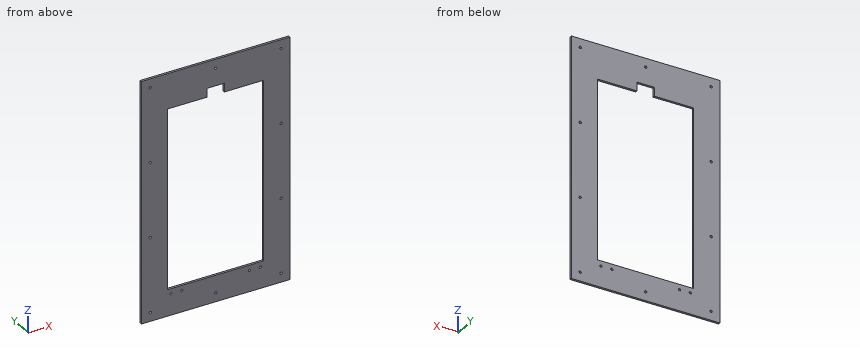
Autodesk Inventor part; units mm, degrees
ref_plane "YZ Plane" through (0, 0, 0) normal (1, 0, 0) x (0, 1, 0)
ref_plane "XZ Plane" through (0, 0, 0) normal (0, 1, 0) x (-1, 0, 0)
ref_plane "XY Plane" through (0, 0, 0) normal (0, 0, 1) x (1, 0, 0)
sketch "Sketch1" plane through (0, 0, 0) normal (0, 1, 0) x (-1, 0, 0)
  line L0 (107.95, -174.625) -> (-107.95, -174.625)
  line L1 (-107.95, -174.625) -> (-107.95, 174.625)
  line L2 (-107.95, 174.625) -> (107.95, 174.625)
  line L3 (107.95, 174.625) -> (107.95, -174.625)
  line L4 (107.95, -174.625) -> (-107.95, 174.625) construction
  line L5 (-107.95, -174.625) -> (107.95, 174.625) construction
  point P0 (0, 0)
  dimension "d0" = 215.9
  dimension "d1" = 349.25
extrude "Thickness" add sketch "Sketch1" along normal blind 3.175
sketch "Cutout Sketch" plane through (0, 3.175, 0) normal (0, 1, 0) x (1, 0, 0)
  line L0 (107.95, -174.625) -> (107.95, 174.625)
  line L1 (107.95, 174.625) -> (-107.95, 174.625)
  line L2 (-107.95, 174.625) -> (-107.95, -174.625)
  line L3 (-107.95, -174.625) -> (107.95, -174.625)
  line L4 (-69.85, 136.525) -> (69.85, 136.525)
  line L5 (69.85, 136.525) -> (69.85, -123.825)
  line L6 (69.85, -123.825) -> (-69.85, -123.825)
  line L7 (-69.85, -123.825) -> (-69.85, 136.525)
  point P0 (0, 0)
  dimension "d4" = 38.1
  dimension "d8" = 38.1
  dimension "d9" = 50.8
  dimension "d10" = 38.1
extrude "Cutout" cut sketch "Cutout Sketch" against normal blind 25.4 contours L4 L5 L6 L7
sketch "Sketch3" plane through (0, 3.175, 0) normal (0, 1, 0) x (1, 0, 0)
  line L0 (69.85, 136.525) -> (69.85, -123.825)
  line L1 (69.85, -123.825) -> (-69.85, -123.825)
  line L2 (-69.85, -123.825) -> (-69.85, 136.525)
  line L3 (-69.85, 136.525) -> (69.85, 136.525)
  line L4 (107.95, 174.625) -> (-107.95, 174.625)
  line L5 (-107.95, 174.625) -> (-107.95, -174.625)
  line L6 (-107.95, -174.625) -> (107.95, -174.625)
  line L7 (107.95, -174.625) -> (107.95, 174.625)
  line L8 (12.7, -136.525) -> (-12.7, -136.525)
  line L9 (-12.7, -136.525) -> (-12.7, -123.825)
  line L10 (-12.7, -123.825) -> (12.7, -123.825)
  line L11 (12.7, -123.825) -> (12.7, -136.525)
  point P0 (0, 0)
  point P1 (0, -136.525)
  point P2 (0, -123.825)
  dimension "d11" = 25.4
  dimension "d12" = 12.7
extrude "Extrusion3" cut sketch "Sketch3" against normal blind 25.4 contours L11 L8 L9 L1
sketch "Sketch4" plane through (0, 3.175, 0) normal (0, 1, 0) x (1, 0, 0)
  circle A0 centre (-65.0875, 144.0656) radius 1.75
  circle A1 centre (65.0875, 144.0656) radius 1.75
  circle A2 centre (49.2125, 144.0656) radius 1.75
  circle A3 centre (-49.2125, 144.0656) radius 1.75
  line L0 (-82.55, 136.525) -> (82.55, 136.525)
  line L1 (82.55, 136.525) -> (82.55, -136.525)
  line L2 (82.55, -136.525) -> (-82.55, -136.525)
  line L3 (-82.55, -136.525) -> (-82.55, 136.525)
  line L4 (107.95, 174.625) -> (-107.95, 174.625)
  line L5 (-107.95, 174.625) -> (-107.95, -174.625)
  line L6 (-107.95, -174.625) -> (107.95, -174.625)
  line L7 (107.95, -174.625) -> (107.95, 174.625)
  circle A4 centre (-95.25, -53.975) radius 1.75
  circle A5 centre (0, -161.925) radius 1.75
  circle A6 centre (95.25, -53.975) radius 1.75
  circle A7 centre (95.25, -161.925) radius 1.75
  circle A8 centre (-95.25, -161.925) radius 1.75
  circle A9 centre (-95.25, 161.925) radius 1.75
  circle A10 centre (95.25, 161.925) radius 1.75
  circle A11 centre (95.25, 53.975) radius 1.75
  circle A12 centre (0, 161.925) radius 1.75
  circle A13 centre (-95.25, 53.975) radius 1.75
  point P0 (0, 0)
hole "Hole1" at (65.0875, 3.175, -144.0656) at (49.2125, 3.175, -144.0656) at (-49.2125, 3.175, -144.0656) at (-65.0875, 3.175, -144.0656) direction (0, -1, 0) diameter 3.5 end through all
sketch "Sketch5" plane through (0, 3.175, 0) normal (0, 1, 0) x (1, 0, 0)
  circle A0 centre (-95.25, -53.975) radius 1.75
  circle A1 centre (0, -161.925) radius 1.75
  circle A2 centre (95.25, -53.975) radius 1.75
  circle A3 centre (95.25, -161.925) radius 1.75
  circle A4 centre (-95.25, -161.925) radius 1.75
  circle A5 centre (-95.25, 161.925) radius 1.75
  circle A6 centre (95.25, 161.925) radius 1.75
  circle A7 centre (95.25, 53.975) radius 1.75
  circle A8 centre (0, 161.925) radius 1.75
  circle A9 centre (-95.25, 53.975) radius 1.75
  circle A10 centre (-65.0875, 144.0656) radius 1.75
  circle A11 centre (65.0875, 144.0656) radius 1.75
  circle A12 centre (49.2125, 144.0656) radius 1.75
  circle A13 centre (-49.2125, 144.0656) radius 1.75
  line L0 (-82.55, 136.525) -> (82.55, 136.525)
  line L1 (82.55, 136.525) -> (82.55, -136.525)
  line L2 (82.55, -136.525) -> (-82.55, -136.525)
  line L3 (-82.55, -136.525) -> (-82.55, 136.525)
  line L4 (107.95, 174.625) -> (-107.95, 174.625)
  line L5 (-107.95, 174.625) -> (-107.95, -174.625)
  line L6 (-107.95, -174.625) -> (107.95, -174.625)
  line L7 (107.95, -174.625) -> (107.95, 174.625)
  point P0 (0, 0)
hole "Hole2" at (-95.25, 3.175, 161.925) at (0, 3.175, 161.925) at (95.25, 3.175, 161.925) at (95.25, 3.175, 53.975) at (95.25, 3.175, -53.975) at (95.25, 3.175, -161.925) at (0, 3.175, -161.925) at (-95.25, 3.175, -161.925) at (-95.25, 3.175, -53.975) at (-95.25, 3.175, 53.975) direction (0, -1, 0) diameter 3.5 end through all
properties part number "NASA-20-EBOX-T" material "Polycarbonate, Clear"
Can you work these out from the model? Positions are in its coordinate system, mm. Round coordinates to 2 decimals unless told otherwise and drop trailing zeros. Loops run counter-clockwise (first coordinate to the right, second up) from the corner with the lowest first, then second, coordinate; pieces in that order, holes last.
Item 1: Suppose I cut it at B-B, the plane x = 24. Write out the boundary of the cut face in (y, z) (3 decimals).
Item 2: Will these pins go through, and if not, where does the flat tip stop? pin 1 Ø2 at (x, z) = (-65.09, -144.07) entering from -Y; pin 2 Ø4.5 at (x, z) = (-95.25, -161.925) entering from +Y (3 decimals).
Item 3: Please list where these lines run through material, in increasing order: L1, parallel to Z at x = -95.25, y = 1.8 (3 decimals); L2, parallel to Z at x = 0, y = 1.65 (3 decimals); L3, parallel to Z at x = -10, y = 1.75 (3 decimals).
Item 4: Suppose I cut it at C-C, the plane y = 1.1. State how many separate pieces and enclosed holes the cut face has, then the cut area to 3 significant figures.
Item 5: Suppose I cut it at A-A, the plane z = -77. Write out the boundary of the cut face in (x, y) (3 decimals), then the cut area to 3 significant figures.
Reported:
1. outline: (0, -174.625) - (3.175, -174.625) - (3.175, -136.525) - (0, -136.525) - close; (0, 123.825) - (3.175, 123.825) - (3.175, 174.625) - (0, 174.625) - close
2. pin 1: passes through
2. pin 2: stops at y = 3.175
3. L1: z = -174.625 to -163.675, -160.175 to -55.725, -52.225 to 52.225, 55.725 to 160.175, 163.675 to 174.625
3. L2: z = -174.625 to -163.675, -160.175 to -136.525, 136.525 to 160.175, 163.675 to 174.625
3. L3: z = -174.625 to -136.525, 136.525 to 174.625
4. separate pieces: 1
4. enclosed holes: 15
4. area: 38,600 mm2
5. outline: (-107.95, 0) - (-69.85, 0) - (-69.85, 3.175) - (-107.95, 3.175) - close; (69.85, 0) - (107.95, 0) - (107.95, 3.175) - (69.85, 3.175) - close
5. area: 242 mm2
